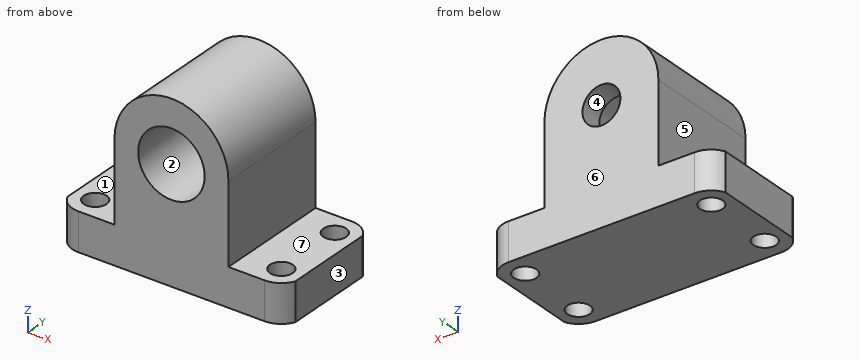
Autodesk Fusion 360 part; units mm, degrees
sketch "Sketch1" plane through (0, 0, 0) normal (0, 0, 1) x (1, 0, 0)
  line L0 (0, 0) -> (-120, 0)
  line L1 (-120, 0) -> (-120, 62)
  line L2 (-120, 62) -> (0, 62)
  line L3 (0, 62) -> (0, 0)
  line L4 (-120, 0) -> (-109, 0)
  line L5 (-120, 62) -> (-109, 62)
  line L6 (0, 62) -> (-11, 62)
  line L7 (0, 0) -> (-11, 0)
  line L8 (-120, 62) -> (-120, 50)
  line L9 (-120, 0) -> (-120, 12)
  line L10 (0, 62) -> (0, 50)
  line L11 (0, 0) -> (0, 12)
  circle A0 centre (-109, 12) radius 6
  circle A1 centre (-109, 12) radius 12
  circle A2 centre (-109, 50) radius 6
  circle A3 centre (-109, 50) radius 12
  circle A4 centre (-11, 50) radius 6
  line L12 (-11, 50) -> (-11, 50.4247)
  circle A5 centre (-11, 50) radius 12
  circle A6 centre (-11, 12) radius 6
  circle A7 centre (-11, 12) radius 12
  dimension "d1" = 120
  dimension "d2" = 62
  dimension "d3" = 11
  dimension "d4" = 11
  dimension "d5" = 11
  dimension "d6" = 11
  dimension "d7" = 12
  dimension "d8" = 12
  dimension "d9" = 12
  dimension "d10" = 12
  dimension "d11" = 12
  dimension "d12" = 24
  dimension "d13" = 12
  dimension "d14" = 24
  dimension "d15" = 12
  dimension "d16" = 24
  dimension "d17" = 12
  dimension "d18" = 24
extrude "Extrude1" add sketch "Sketch1" along normal blind 20 contours L0 L1 L2 L3 A1 A3 A5 A7 | L3 L11 A7 | L1 L9 A1 | L3 L10 A5 | L1 L8 A3 picked at (-1.7555, 9.8119) picked at (-118.2445, 14.1881) picked at (-1.7555, 52.1881) picked at (-118.2445, 47.8119)
sketch "Sketch2" plane through (0, 0, 0) normal (0, -1, 0) x (1, 0, 0)
  line L0 (-109, 0) -> (-11, 0)
  line L1 (-11, 0) -> (-11, 20)
  line L2 (-11, 20) -> (-109, 20)
  line L3 (-109, 20) -> (-109, 0)
  line L4 (-109, 20) -> (-11, 20)
  line L5 (-60, 20) -> (-90, 20)
  line L6 (-60, 20) -> (-30, 20)
  line L7 (-90, 20) -> (-90, 62)
  line L8 (-30, 20) -> (-30, 62)
  line L9 (-90, 62) -> (-30, 62)
  dimension "d21" = 30
  dimension "d22" = 30
  dimension "d23" = 42
  dimension "d24" = 42
extrude "Extrude2" add sketch "Sketch2" against normal blind 62 contours L2 L4 L5 L6 L7 L8 L9
sketch "Sketch3" plane through (0, 0, 0) normal (0, -1, 0) x (1, 0, 0)
  line L0 (-109, 0) -> (-11, 0)
  line L1 (-11, 0) -> (-11, 20)
  line L2 (-11, 20) -> (-30, 20)
  line L3 (-30, 20) -> (-30, 62)
  line L4 (-30, 62) -> (-90, 62)
  line L5 (-90, 62) -> (-90, 20)
  line L6 (-90, 20) -> (-109, 20)
  line L7 (-109, 20) -> (-109, 0)
  circle A0 centre (-60, 62) radius 30
  line L8 (-90, 62) -> (-30, 62)
extrude "Extrude3" add sketch "Sketch3" against normal blind 62 contours L4 A0 L8 picked at (-62.2252, 71.7493)
sketch "Sketch4" plane through (0, 0, 0) normal (0, -1, 0) x (1, 0, 0)
  line L0 (-109, 0) -> (-11, 0)
  line L1 (-11, 0) -> (-11, 20)
  line L2 (-11, 20) -> (-30, 20)
  line L3 (-30, 20) -> (-30, 62)
  arc A0 (-30, 62) -> (-90, 62) centre (-60, 62) ccw
  line L4 (-90, 62) -> (-90, 20)
  line L5 (-90, 20) -> (-109, 20)
  line L6 (-109, 20) -> (-109, 0)
  circle A1 centre (-60, 59.9304) radius 17.5
  dimension "d29" = 35
extrude "Extrude4" cut sketch "Sketch4" against normal blind 50 contours A1
sketch "Sketch5" plane through (0, 50, 0) normal (0, -1, 0) x (1, 0, 0)
  circle A0 centre (-60, 59.9304) radius 17.5
  circle A1 centre (-60, 59.9304) radius 10
  dimension "d32" = 20
extrude "Extrude5" cut sketch "Sketch5" against normal blind 35 contours A1
sketch "Sketch6" plane through (0, 0, 0) normal (0, 0, -1) x (1, 0, 0)
  circle A0 centre (-109, -12) radius 6
  circle A1 centre (-11, -12) radius 6
  circle A2 centre (-11, -50) radius 6
  circle A3 centre (-109, -50) radius 6
  arc A4 (-11, -62) -> (0, -54.7958) centre (-11, -50) ccw
  line L0 (0, -54.7958) -> (0, -7.2042)
  arc A5 (0, -7.2042) -> (-11, 0) centre (-11, -12) ccw
  line L1 (-11, 0) -> (-109, 0)
  arc A6 (-109, 0) -> (-120, -7.2042) centre (-109, -12) ccw
  line L2 (-120, -7.2042) -> (-120, -54.7958)
  arc A7 (-120, -54.7958) -> (-109, -62) centre (-109, -50) ccw
  line L3 (-109, -62) -> (-11, -62)
Design review of the part built by this model. Coordinates are the model's own, in mm. Face numbers are marked on the shaded views. A direction names the side the tool comes from. Round coordinates to 2 decimals unless told otherwise and drop trailing zeros. Write each loop counter-clockwise with the first axis right and the second up, starting at its lowest first coordinate (ties: lowest second). Pieces come first, ordered by that corner, then holes. Notation, with made-up numbers: (-40, 21) -> (-13, 21) arc R20 cw to (-13, 60) -> close; hole circle Ø5 at (78.25, 25). An arc over 180 degrees is marked (long way). Write item = value, one per line. Start each with the question number.
1) Take a section at B-B, the plane y = 16. State the section outline as (x, z) points.
2) Take a section at D-D, the plane x = -75.5. State the section outline as (y, z) points.
3) Wall thickness on probe 1 along Y at (x, z) = (-109, 13.5); probe 2 along Z at (x, y) = (-60, 56); probe 3 along Z at (x, y) = (-106, 17.5): over which ranges is each line inside the solid? List them lowest first. Write a range as from..to.
4) Take a section at C-C, the plane x = -60. State the section outline as (y, z) points.
5) Tool access review of the marked faces 5, 6 and 7: name each direction out of +Z, -Z, +X, -X, +Y, -Y from which nothing blocks a thin tool from reaching the whole face with its end or side.
6) Take a section at A-A, the plane z = 9. State the section outline as (x, y) points.
7) Mouldability with a two-part tool opening along X and no side actions: class the marked faces 1, 2, 3 and 4 as +X half, -X half, draft (parallel to the pull), parting line (faces both ways), or undercut.
8) Clearance check with flat-ended pins moving along their axes: pin 1 (1.5 mm diameter, centred on y = 24, z = 26, fed in from -X); pin 2 (18 mm diameter, centred on x = -60, z = 59.93, fed in from -Y); pin 3 (1 mm diameter, centred on x = -66.5, y = 32.5, fed in from +Z); pin 4 (10 mm diameter, centred on x = -90, y = 21.5, fed in from +Z). State where each tip first meets the part, or that it passes through.
Results list:
q1.outline = (-120, 0) -> (-113.47, 0) -> (-113.47, 20) -> (-120, 20) -> close; (-104.53, 0) -> (-15.47, 0) -> (-15.47, 20) -> (-30, 20) -> (-30, 62) arc R30 ccw to (-90, 62) -> (-90, 20) -> (-104.53, 20) -> close; (-6.53, 0) -> (0, 0) -> (0, 20) -> (-6.53, 20) -> close; hole circle Ø35 at (-60, 59.93)
q2.outline = (0, 0) -> (62, 0) -> (62, 87.69) -> (0, 87.69) -> (0, 68.05) -> (50, 68.05) -> (50, 51.81) -> (0, 51.81) -> close
q3.probe_1 = 0..6, 18..44, 56..62
q3.probe_2 = 0..49.93, 69.93..92
q3.probe_3 = 0..20
q4.outline = (0, 0) -> (62, 0) -> (62, 49.93) -> (50, 49.93) -> (50, 42.43) -> (0, 42.43) -> close; (0, 77.43) -> (50, 77.43) -> (50, 69.93) -> (62, 69.93) -> (62, 92) -> (0, 92) -> close
q5.face_5 = +Z, -X, +Y, -Y
q5.face_6 = +Z, -Z, +X, -X, +Y
q5.face_7 = +Z, +X, +Y, -Y
q6.outline = (-120, 7.2) arc R12 ccw to (-109, 0) -> (-11, 0) arc R12 ccw to (0, 7.2) -> (0, 54.8) arc R12 ccw to (-11, 62) -> (-109, 62) arc R12 ccw to (-120, 54.8) -> close; hole circle Ø12 at (-109, 12); hole circle Ø12 at (-109, 50); hole circle Ø12 at (-11, 12); hole circle Ø12 at (-11, 50)
q7.face_1 = draft
q7.face_2 = undercut
q7.face_3 = +X half
q7.face_4 = undercut
q8.pin_1 = -90
q8.pin_2 = through
q8.pin_3 = 91.39
q8.pin_4 = 78.58
